Input: part model. Units: mm. Frame: model coordinates. Face numbers are marked on the shaded views. A direction names the side the tool comes from. Give positions to 0.01 mm unless a question says otherwise; leave off trailing zeros. Loops run counter-clockwise (first coordinate to the right, second up) from the corner with the lowest first, then second, coordinate; pieces in that order, holes last. Notation, with made-up numbers: M -30,58 L 2,58 A21 cw 2,94 Z; hole C -8,-2.5 d11. An arc over 180 degrees is marked long. Use a Markdown table: item, result. Add a question column.
from build123d import *

# Parameters (mm, degrees)
SKETCH1_W                = 29
SKETCH1_H                = 15.5
BOSS_EXTRUDE1_DEPTH      = 8
SHELL1_T                 = -1
SKETCH2_W                = 1
SKETCH2_H                = 13.5
BOSS_EXTRUDE2_DEPTH      = 7
SKETCH3_W                = 8
SKETCH3_H                = 3
CUT_EXTRUDE1_DEPTH       = 7
SKETCH4_W                = 29
SKETCH4_H                = 2
BOSS_EXTRUDE3_DEPTH      = 15.5
INTERSECT1_OUTLINE_W     = 29
INTERSECT1_OUTLINE_H     = 15.5
INTERSECT1_OUTLINE_W_2   = 8
INTERSECT1_OUTLINE_H_2   = 3
INTERSECT1_DEPTH         = 7
INTERSECT1_START         = 7
INTERSECT1_2_OUTLINE_W   = 29
INTERSECT1_2_OUTLINE_H   = 15.5
INTERSECT1_2_OUTLINE_W_2 = 13
INTERSECT1_2_OUTLINE_H_2 = 13.5
INTERSECT1_2_DEPTH       = 1
SKETCH5_W                = 8
SKETCH5_H                = 8
CUT_EXTRUDE2_DEPTH       = 15.5


# Read off the part's stored shape, not the designer's step: Intersect1
with BuildPart() as part:
    # Sketch1 → Boss-Extrude1 (new body)
    with BuildSketch(Plane(origin=(0, 0, 0), x_dir=(1, 0, 0), z_dir=(0, 1, 0))):
        Rectangle(SKETCH1_W, SKETCH1_H)
    extrude(amount=BOSS_EXTRUDE1_DEPTH)

    # Shell1
    shell1_openings = [part.faces().sort_by_distance(p)[0] for p in [
        (0, 8, 0),
    ]]
    offset(amount=SHELL1_T, openings=shell1_openings, kind=Kind.INTERSECTION)

    # Sketch2 → Boss-Extrude2 (add)
    with BuildSketch(Plane(origin=(0, 1, 0), x_dir=(1, 0, 0), z_dir=(0, 1, 0))):
        Rectangle(SKETCH2_W, SKETCH2_H)
    extrude(amount=BOSS_EXTRUDE2_DEPTH)

    # Sketch3 → Cut-Extrude1 (cut)
    with BuildSketch(Plane(origin=(0, 1, 0), x_dir=(1, 0, 0), z_dir=(0, 1, 0))):
        with Locations((-7.25, 5.25)):
            Rectangle(SKETCH3_W, SKETCH3_H)
        with Locations((7.25, 5.25)):
            Rectangle(SKETCH3_W, SKETCH3_H)
        with Locations((7.25, -5.25)):
            Rectangle(SKETCH3_W, SKETCH3_H)
        with Locations((-7.25, -5.25)):
            Rectangle(SKETCH3_W, SKETCH3_H)
    extrude(amount=-CUT_EXTRUDE1_DEPTH, mode=Mode.SUBTRACT)

    # Intersect1 outline → Intersect1 (cut)
    with BuildSketch(Plane(origin=(0, 0, 0), x_dir=(1, 0, 0), z_dir=(0, 1, 0))):
        Rectangle(INTERSECT1_OUTLINE_W, INTERSECT1_OUTLINE_H)
        with Locations((-7.25, -5.25)):
            Rectangle(INTERSECT1_OUTLINE_W_2, INTERSECT1_OUTLINE_H_2, mode=Mode.SUBTRACT)
        with Locations((-7.25, 5.25)):
            Rectangle(INTERSECT1_OUTLINE_W_2, INTERSECT1_OUTLINE_H_2, mode=Mode.SUBTRACT)
        with Locations((7.25, 5.25)):
            Rectangle(INTERSECT1_OUTLINE_W_2, INTERSECT1_OUTLINE_H_2, mode=Mode.SUBTRACT)
        with Locations((7.25, -5.25)):
            Rectangle(INTERSECT1_OUTLINE_W_2, INTERSECT1_OUTLINE_H_2, mode=Mode.SUBTRACT)
    extrude(amount=INTERSECT1_DEPTH, mode=Mode.SUBTRACT)


with BuildPart() as body_2:
    # Sketch4 → Boss-Extrude3 (new body)
    with BuildSketch(Plane.XY.offset(7.75)):
        with Locations((0, 8)):
            Rectangle(SKETCH4_W, SKETCH4_H)
    extrude(amount=-BOSS_EXTRUDE3_DEPTH)


with BuildPart() as intersect1_2_tool:
    # Intersect1 2 outline → Intersect1 2 (new body)
    with BuildSketch(Plane(origin=(0, 0, 0), x_dir=(1, 0, 0), z_dir=(0, 1, 0)).offset(INTERSECT1_START)):
        Rectangle(INTERSECT1_2_OUTLINE_W, INTERSECT1_2_OUTLINE_H)
        with Locations((-7, 0)):
            Rectangle(INTERSECT1_2_OUTLINE_W_2, INTERSECT1_2_OUTLINE_H_2, mode=Mode.SUBTRACT)
        with Locations((7, 0)):
            Rectangle(INTERSECT1_2_OUTLINE_W_2, INTERSECT1_2_OUTLINE_H_2, mode=Mode.SUBTRACT)
    extrude(amount=INTERSECT1_2_DEPTH)


with BuildPart() as part_1:
    add(part.part)

    # Intersect1 2: cut by intersect1_2_tool
    add(intersect1_2_tool.part, mode=Mode.SUBTRACT)


with BuildPart() as body_2_1:
    add(body_2.part)

    # Intersect1 2: cut by intersect1_2_tool
    add(intersect1_2_tool.part, mode=Mode.SUBTRACT)

    # Sketch5 → Cut-Extrude2 (cut)
    with BuildSketch(Plane(origin=(0, 9, 0), x_dir=(1, 0, 0), z_dir=(0, 1, 0))):
        with Locations((-7.25, 0)):
            Rectangle(SKETCH5_W, SKETCH5_H)
        with Locations((7.25, 0)):
            Rectangle(SKETCH5_W, SKETCH5_H)
    extrude(amount=-CUT_EXTRUDE2_DEPTH, mode=Mode.SUBTRACT)


solid = body_2_1.part
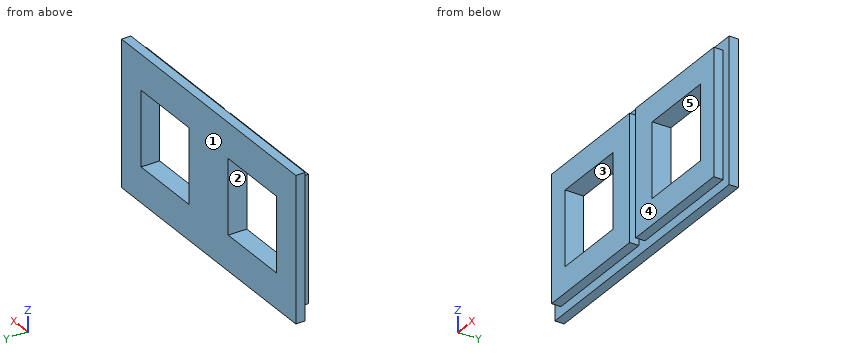
1) Section query C-C, the plane z = 2. Return the cut outline in (x, y), and give its area (3 significant figures).
2) Section query B-B, the plane x = -8.25. Return the cut outline in (y, z), and give its area (3 significant figures).
3) Pull-direction query (Z, two-part tool) for the marked faces 1, 2 and 3; classes: pulls with the +Z half, pulls with the -Z half, needs draft (parallel to the pull), parting line crosses it, or undercut.
4) Contact query for flat-ended pins moving along their axis: P1, Ø0.8, axis at x = -4.5, y = 7.5, coming from the +Z side; P2, Ø0.5, axis at y = 7.5, z = 2, coming from the +X side; P3, Ø0.8, axis at y = 7.5, z = 0.5, coming from the -X side. Output: stop coordinate, or through.
5) Ray query, line 1 (X direction, y = 7.75, z = 0); line 2 (X direction, y = 8.85, z = -3.25); line 3 (X direction, y = 7.1, z = 5.75). Return the intervals inside material, ascending. Write a range as [from, to].
6) Section query D-D, the plane z = 5. Return the cut outline in (x, y).
7) Reachability of the marked faces 4 and 5 from +Z, -Z, +X, -X, +Y, -Y: full face, straight path, thin tool, end or side. Return the list, or none.
8) Section query A-A, the plane y = 7.4. Return the cut outline in (x, z).
Entries:
| question | item | result |
|---|---|---|
| 1 | outline | M -14.5,8 L -13.5,8 L -13.5,7 L -11.25,7 L -11.25,9 L -14.5,9 Z; M -3.25,7 L -0.5,7 L -0.5,8 L 0.5,8 L 0.5,7 L 3.25,7 L 3.25,9 L -3.25,9 Z; M 11.25,7 L 13.5,7 L 13.5,8 L 14.5,8 L 14.5,9 L 11.25,9 Z |
| 1 | area | 23.0 mm² |
| 2 | outline | M 7,-6.75 L 8,-6.75 L 8,-7.75 L 9,-7.75 L 9,-4 L 7,-4 Z; M 7,4 L 9,4 L 9,7.75 L 8,7.75 L 8,6.75 L 7,6.75 Z |
| 2 | area | 13.0 mm² |
| 3 | face 1 | needs draft |
| 3 | face 2 | undercut |
| 3 | face 3 | undercut |
| 4 | P1 | stops at z = 6.75 |
| 4 | P2 | stops at x = 13.5 |
| 4 | P3 | stops at x = -13.5 |
| 5 | line 1 | x = [-13.5, -11.25], [-3.25, -0.5], [0.5, 3.25], [11.25, 13.5] |
| 5 | line 2 | x = [-14.5, -11.25], [-3.25, 3.25], [11.25, 14.5] |
| 5 | line 3 | x = [-13.5, -0.5], [0.5, 13.5] |
| 6 | outline | M -14.5,8 L -13.5,8 L -13.5,7 L -0.5,7 L -0.5,8 L 0.5,8 L 0.5,7 L 13.5,7 L 13.5,8 L 14.5,8 L 14.5,9 L -14.5,9 Z |
| 7 | face 4 | +Z, -Z, +X, -X, -Y |
| 7 | face 5 | +Y, -Y |
| 8 | outline | M -13.5,-6.75 L -0.5,-6.75 L -0.5,6.75 L -13.5,6.75 Z; M 0.5,-6.75 L 13.5,-6.75 L 13.5,6.75 L 0.5,6.75 Z; hole M -11.25,-4 L -3.25,-4 L -3.25,4 L -11.25,4 Z; hole M 3.25,-4 L 11.25,-4 L 11.25,4 L 3.25,4 Z |
